Geometry check sheet. Reference: the model listing, model coordinates, mm. A direction names the side the tool comes from. Round coordinates to 2 decimals unless told otherwise and drop trailing zeros. Order: outer loops, then holes, each group sorted by start corner. A loop starts at its lowest first (then second) coordinate and runs counter-clockwise, first axis right, second up. Notation, with made-up numbers: (-21, 35.5) -> (2, 35.5) arc R26 ccw to (2, 73.5) -> close; hole circle Ø8 at (-13, -4). An arc over 180 degrees is marked (long way). Answer as a JSON object with one key per item and string values. Group by question number.
from build123d import *

# Parameters (mm, degrees)
SKETCH1_W           = 25.4
SKETCH1_H           = 152.4
BOSS_EXTRUDE1_DEPTH = 3.18
CUT_EXTRUDE1_DEPTH  = 3.18


with BuildPart() as part:
    # Sketch1 → Boss-Extrude1 (new body)
    with BuildSketch(Plane(origin=(0, 0, 0), x_dir=(1, 0, 0), z_dir=(0, 1, 0))):
        Rectangle(SKETCH1_W, SKETCH1_H)
    extrude(amount=BOSS_EXTRUDE1_DEPTH)

    # Sketch2 → Cut-Extrude1 (cut)
    with BuildSketch(Plane(origin=(0, 3.18, 0), x_dir=(1, 0, 0), z_dir=(0, 1, 0))):
        Polygon((-1.59, 73.02), (-1.59, 70.02), (-2.5, 70.02), (-2.5, 68.02), (-1.59, 68.02), (-1.59, 64.2), (0, 64.2), (1.59, 64.2), (1.59, 68.02), (2.5, 68.02), (2.5, 70.02), (1.59, 70.02), (1.59, 73.02), (5, 73.02), (5, 76.2), (-5, 76.2), (-5, 73.02), align=None)
        Polygon((0, -64.2), (-1.59, -64.2), (-1.59, -68.02), (-2.5, -68.02), (-2.5, -70.02), (-1.59, -70.02), (-1.59, -73.02), (-5, -73.02), (-5, -76.2), (5, -76.2), (5, -73.02), (1.59, -73.02), (1.59, -70.02), (2.5, -70.02), (2.5, -68.02), (1.59, -68.02), (1.59, -64.2), align=None)
    extrude(amount=-CUT_EXTRUDE1_DEPTH, mode=Mode.SUBTRACT)


solid = part.part
Item 1: Thickness scan on L1, parallel to Z at x = 2, y = 0.25; L2, parallel to X at y = 1.6, z = 66; L3, parallel to Z at x = -4.75, y = 2.85. Record the ranges inside material, lowest first.
Item 2: Set-up check for faces 1 (the flat face through (0, 2, 64.2)), 2 (the flat face through (-9, 2, -76.2)), 3 (the flat face through (-1.59, 2, -72)): record each of +Z, -Z, +X, -X, +Y, -Y from which the full face is reachable in a straight line by a thin tool's end or side.
Item 3: Depth check by flat-ended pin: pin 1 Ø1.6 at (x, y) = (2.5, 1.5) entering from +Z; pin 2 Ø1 at (x, y) = (4, 1) entering from -Z. Enter the tip coordinate at first touch or a pass-through.
Item 4: Mould release check, pull along X, two halves, no side actions. Record for faces 4 (the flat face through (12.7, 2, 1)), 5 (the flat face through (-12.7, 2, 1)), 6 (the flat face through (-9, 2, 76.2)), 7 (the flat face through (1.59, 2, -71)): pulls with the +X half, pulls with the -X half, needs draft (parallel to the pull), parting line crosses it, or undercut.
Item 5: Sectioned sample at A-A, the plane x = 0. Enter the section's corners in (y, z), then the cut area to 3 significant figures.
Result:
{
 "1": {"L1": "z = -73.02 to -70.02, -68.02 to 68.02, 70.02 to 73.02", "L2": "x = -12.7 to -1.59, 1.59 to 12.7", "L3": "z = -73.02 to 73.02"},
 "2": {"face 1": "+Z, +Y, -Y", "face 2": "-Z, +X, -X, +Y, -Y", "face 3": "-Z, +Y, -Y"},
 "3": {"pin 1": "stops at z = 73.02", "pin 2": "stops at z = -73.02"},
 "4": {"face 4": "pulls with the +X half", "face 5": "pulls with the -X half", "face 6": "needs draft", "face 7": "undercut"},
 "5": {"outline": "(0, -64.2) -> (3.18, -64.2) -> (3.18, 64.2) -> (0, 64.2) -> close", "area": "408 mm2"}
}
